Read the model definition and answer for the solid it produces. Units are mm, in the model's axes. A direction names the side the tool comes from. Coordinates: 2 decimals unless noted, no trailing zeros. Loops run counter-clockwise (first coordinate to the right, second up) from the corner with the lowest first, then second, coordinate; pieces in that order, holes last. Notation, with made-up numbers: (-36.75, 88.25) -> (8.25, 88.25) arc R11 cw to (8.25, 100.25) -> close; hole circle Ø9 at (24, 7.5). An arc over 180 degrees is marked (long way). Answer as a JSON object with one key per item and string values. Group by question number.
Q1. Determine the mould class of faces 4 (the flat face through (0, 0, 2)), 5 (the cylindrical face through (0.16, 13.14, 0.99)), 6 (the flat face through (8.35, 10, 1)) for opening direction Y: released by +Y, released by -Y, zero draft, split by the parting line, or undercut.
Q2. The part is cut by section C-C on y = -10. Write down the section's boundary in (x, z).
Q3. Each of these flat-tipped pins is pushed along its axis until it touches: P1, Ø0.6, axis at x = 9.5, z = 0.5, coming from the +Y side; P2, Ø0.6, axis at y = -10, z = 0.5, coming from the +X side; P3, Ø1, axis at x = 9, z = 1, coming from the -Y side. Where does it stop, or does it pass through?
Q4. For faces 1 (the flat face through (-11.35, 0, 1)), 2 (the flat face through (-9, -8.875, 1)), 3 (the flat face through (8.35, -10, 1)), determine the directions among +Z, -Z, +X, -X, +Y, -Y from which every point of the face is accessible in a straight line to the end or side of a thin tool.
Q5. The part is cut by section D-D on x = -6. Write down the section's boundary in (y, z).
Q6. Straight lines are drawn through the part: line 1 along X through (y, z) = (-10, 0.5); line 2 along Y through (x, z) = (-2.5, 1.7); line 3 along Y through (x, z) = (-6, 1.2). For each, find the intervals that lie inside material, in ascending order. Write a range as [from, to].
Q7. The part is cut by section B-B on x = -9.5. Write down the section's boundary in (y, z) (3 decimals).
from build123d import *

# Parameters (mm, degrees)
EXTRUDE_1_DEPTH = 2


with BuildPart() as part:
    # 草图1 → 凸台-拉伸1 (new body)
    with BuildSketch(Plane.XY):
        with BuildLine():
            Line((8.35, 10.875), (11.28, 10.875))
            ThreePointArc((11.28, 10.875), (11.329497475, 10.895502525), (11.35, 10.945))
            Line((11.35, 10.945), (11.35, 11.445))
            ThreePointArc((11.35, 11.445), (11.336054538, 11.486927185), (11.299774606, 11.512148827))
            ThreePointArc((11.299774606, 11.512148827), (0, 13.14139051), (-11.299774606, 11.512148827))
            ThreePointArc((-11.299774606, 11.512148827), (-11.336054538, 11.486927185), (-11.35, 11.445))
            Line((-11.35, 11.445), (-11.35, 10.945))
            ThreePointArc((-11.35, 10.945), (-11.329497475, 10.895502525), (-11.28, 10.875))
            Line((-11.28, 10.875), (-8.35, 10.875))
            Line((-8.35, 10.875), (-8.35, 8.875))
            Line((-8.35, 8.875), (-10.591620109, 8.875))
            ThreePointArc((-10.591620109, 8.875), (-11.127875673, 8.652875673), (-11.35, 8.116620109))
            Line((-11.35, 8.116620109), (-11.35, -8.116620109))
            ThreePointArc((-11.35, -8.116620109), (-11.127875673, -8.652875673), (-10.591620109, -8.875))
            Line((-10.591620109, -8.875), (-8.35, -8.875))
            Line((-8.35, -8.875), (-8.35, -10.875))
            Line((-8.35, -10.875), (-11.28, -10.875))
            ThreePointArc((-11.28, -10.875), (-11.329497475, -10.895502525), (-11.35, -10.945))
            Line((-11.35, -10.945), (-11.35, -11.445))
            ThreePointArc((-11.35, -11.445), (-11.336054538, -11.486927185), (-11.299774606, -11.512148827))
            ThreePointArc((-11.299774606, -11.512148827), (0, -13.14139051), (11.299774606, -11.512148827))
            ThreePointArc((11.299774606, -11.512148827), (11.336054538, -11.486927185), (11.35, -11.445))
            Line((11.35, -11.445), (11.35, -10.945))
            ThreePointArc((11.35, -10.945), (11.329497475, -10.895502525), (11.28, -10.875))
            Line((11.28, -10.875), (8.35, -10.875))
            Line((8.35, -10.875), (8.35, -8.875))
            Line((8.35, -8.875), (10.591620109, -8.875))
            ThreePointArc((10.591620109, -8.875), (11.127875673, -8.652875673), (11.35, -8.116620109))
            Line((11.35, -8.116620109), (11.35, 8.116620109))
            ThreePointArc((11.35, 8.116620109), (11.127875673, 8.652875673), (10.591620109, 8.875))
            Line((10.591620109, 8.875), (8.35, 8.875))
            Line((8.35, 8.875), (8.35, 10.875))
        make_face()
    extrude(amount=EXTRUDE_1_DEPTH)


solid = part.part
Final values:
{
 "1": {"face 4": "zero draft", "face 5": "released by +Y", "face 6": "undercut"},
 "2": {"outline": "(-8.35, 0) -> (8.35, 0) -> (8.35, 2) -> (-8.35, 2) -> close"},
 "3": {"P1": "stops at y = 12.07", "P2": "stops at x = 8.35", "P3": "stops at y = -12.23"},
 "4": {"face 1": "+Z, -Z, -X, +Y, -Y", "face 2": "+Z, -Z, -X", "face 3": "+Z, -Z, +X"},
 "5": {"outline": "(-12.69, 0) -> (12.69, 0) -> (12.69, 2) -> (-12.69, 2) -> close"},
 "6": {"line 1": "x = [-8.35, 8.35]", "line 2": "y = [-13.06, 13.06]", "line 3": "y = [-12.69, 12.69]"},
 "7": {"outline": "(-11.997, 0) -> (-10.875, 0) -> (-10.875, 2) -> (-11.997, 2) -> close; (-8.875, 0) -> (8.875, 0) -> (8.875, 2) -> (-8.875, 2) -> close; (10.875, 0) -> (11.997, 0) -> (11.997, 2) -> (10.875, 2) -> close"}
}
